Autodesk Inventor part; units mm, degrees
ref_plane "YZ Plane" through (0, 0, 0) normal (1, 0, 0) x (0, 1, 0)
ref_plane "XZ Plane" through (0, 0, 0) normal (0, 1, 0) x (-1, 0, 0)
ref_plane "XY Plane" through (0, 0, 0) normal (0, 0, 1) x (1, 0, 0)
sketch "Sketch1" plane through (0, 0, 0) normal (1, 0, 0) x (0, 1, 0)
  line L0 (0, 0) -> (64, 0)
  line L1 (0, 0) -> (56, 0)
  line L2 (0, 0) -> (8, 0)
  line L3 (0, 0) -> (0, -95)
  line L4 (0, 0) -> (0, -82)
  line L5 (0, 0) -> (6, 0)
  line L6 (64, 0) -> (64, -13)
  line L7 (64, -13) -> (64, -22)
  line L8 (56, 0) -> (56, -13) construction
  line L9 (56, -22) -> (64, -22) construction
  line L10 (56, -22) -> (56, -95) construction
  line L11 (56, -95) -> (0, -95) construction
  line L12 (64, -22) -> (56, -22)
  line L13 (0, -95) -> (0, -107)
  line L14 (0, -107) -> (8, -107)
  line L15 (8, -107) -> (8, -95)
  line L16 (113.6296, 0) -> (-73.0224, 0)
  line L17 (0, -82) -> (56, -82) construction
  line L18 (8, -95) -> (8, -82)
  line L19 (56, -82) -> (8, -82)
  line L20 (56, -82) -> (56, -22)
  line L21 (8, -95) -> (0, -95)
  arc A0 (0, -85.7011) -> (56, -22) centre (-35.8458, 2.2766) ccw construction
  line L22 (0, -82) -> (0, -85.7011)
  line L23 (56, -22) -> (56, -30)
  line L24 (56, -13) -> (56, 0) construction
  arc A1 (0, -82) -> (54.4542, -13) centre (-35.8458, 2.2766) ccw construction
  line L25 (64, -13) -> (54.4542, -13)
  line L26 (56, -22) -> (56, 0) construction
  arc A2 (8, -82) -> (56, -22) centre (-35.8458, 2.2766) ccw
  line L27 (-35.8458, 2.2766) -> (-35.8458, 0)
  arc A3 (0, -82) -> (54.4542, -13) centre (-35.8458, 2.2766) ccw
  line L28 (8, -82) -> (0, -82)
  point P0 (-35.8458, 1.1383)
  point P1 (8, -82)
  point P2 (8, -82)
  dimension "d0" = 64
  dimension "d1" = 56
  dimension "d2" = 8
  dimension "d3" = 95
  dimension "d4" = 82
  dimension "d5" = 6
  dimension "d6" = 13
  dimension "d7" = 9
  dimension "d12" = 12
ref_plane "Work Plane3" through (0, 0, 0) normal (0, -1, 0) x (1, 0, 0)
sketch "Sketch3" plane through (0, 0, 0) normal (0, -1, 0) x (1, 0, 0)
  circle A0 centre (0, 0) radius 95
  circle A1 centre (0, -95) radius 11.9643
  circle A2 centre (82.2724, -47.5) radius 11.9643
  circle A3 centre (82.2724, 47.5) radius 11.9643
  circle A4 centre (0, 95) radius 11.9643
  circle A5 centre (-82.2724, 47.5) radius 11.9643
  circle A6 centre (-82.2724, -47.5) radius 11.9643
  dimension "d15" = 360
ref_plane "Work Plane1" through (0, 56, 0) normal (0, 1, 0) x (1, 0, 0)
extrude "Extrusion2" add sketch "Sketch3" against normal blind 8 contours A3 A0 | A0 A3 | A2 A0 | A0 A2 | A4 A0 | A0 A4 | A1 A0 | A0 A1 | A5 A0 | A0 A5 | A6 A0 | A0 A6
revolve "Revolution2" add sketch "Sketch1" angle 360 about axis through (0, 113.6296, 0) along (0, -1, 0) contours L0 L6 L25 A3 L3 | L28 L18 L21 L3 | A3 L25 L7 L12 A2 L28 | A2 L20 L19
sketch "Sketch5" plane through (0, 56, 0) normal (0, 1, 0) x (1, 0, 0)
  arc A0 (-75.6497, 57.4641) -> (-87.5902, 36.7825) centre (-82.2724, 47.5) ccw
  circle A1 centre (-82.2724, 47.5) radius 4
  circle A2 centre (-82.2724, -47.5) radius 4
  circle A3 centre (0, -95) radius 4
  circle A4 centre (82.2724, -47.5) radius 4
  circle A5 centre (82.2724, 47.5) radius 4
  circle A6 centre (0, 95) radius 4
  point P0 (0, 0)
  dimension "d20" = 8
  dimension "d23" = 360
extrude "Extrusion3" cut sketch "Sketch5" against normal blind 64
sketch "Sketch8" plane through (0, 64, 0) normal (0, 1, 0) x (1, 0, 0)
  circle A0 centre (0, 0) radius 13
  dimension "d39" = 26
extrude "Extrusion4" cut sketch "Sketch8" against normal blind 64
sketch "Sketch9" plane through (0, 56, 0) normal (0, 1, 0) x (1, 0, 0)
  circle A0 centre (0, 0) radius 82
  line L0 (0, 82) -> (67.9153, 82) construction
  line L1 (0, 82) -> (8, 82)
  line L2 (-82, 0) -> (82, 0)
  line L3 (8, 82) -> (8, 0)
  line L4 (8, 82) -> (-8, 82)
  line L5 (-8, 82) -> (-8, 0)
  line L6 (0, 0) -> (0, -42) construction
  line L7 (0, -42) -> (0, -61) construction
  circle A1 centre (0, -42) radius 12 construction
  circle A2 centre (0, -42) radius 8 construction
  circle A3 centre (0, -61) radius 12 construction
  circle A4 centre (0, -61) radius 8 construction
  line L8 (-12, -61) -> (-12, -42)
  line L9 (12, -61) -> (12, -42)
  line L10 (-12, -61) -> (12, -61) construction
  line L11 (-12, -42) -> (12, -42) construction
  arc A5 (-12, -61) -> (12, -61) centre (0, -61) ccw
  arc A6 (12, -42) -> (-12, -42) centre (0, -42) ccw
  arc A7 (8, -42) -> (-8, -42) centre (0, -42) ccw
  arc A8 (-8, -61) -> (8, -61) centre (0, -61) ccw
  line L12 (-8, -61) -> (-8, -42)
  line L13 (8, -61) -> (8, -42)
  point P0 (8, 81.6088)
  point P1 (-8, 81.6088)
  dimension "d42" = 8
  dimension "d43" = 16
  dimension "d44" = 42
  dimension "d45" = 19
  dimension "d46" = 24
  dimension "d47" = 16
  dimension "d48" = 24
  dimension "d49" = 16
extrude "Extrusion5" cut sketch "Sketch9" against normal blind 56 contours L2 A0 | A0 L5 L2 | L2 L3 A0
revolve "Revolution3" add sketch "Sketch1" angle 360 about axis through (0, 113.6296, 0) along (0, -1, 0) contours A3 L25 L7 L12 A2 L28
sketch "Sketch10" plane through (0, 56, 61) normal (0, 1, 0) x (1, 0, 0)
  circle A0 centre (0, 0) radius 8
  arc A1 (12, 19) -> (-12, 19) centre (0, 19) ccw
  circle A2 centre (0, 19) radius 8
  line L0 (-8, 0) -> (-8, 19)
  line L1 (8, 0) -> (8, 19)
  arc A3 (-12, 0) -> (12, 0) centre (0, 0) ccw
  line L2 (0, 0) -> (0, 19)
  line L3 (-8, 0) -> (8, 0)
  point P0 (0, 61)
  dimension "d54" = 16
  dimension "d55" = 16
extrude "Extrusion6" cut sketch "Sketch10" against normal blind 56
sketch "Sketch11" plane through (8, 56, -20.4939) normal (1, 0, 0) x (0, 0, -1)
  point P0 (-20.4939, -56)
sketch "Sketch12" plane through (0, 56, 0) normal (0, 1, 0) x (1, 0, 0)
  arc A0 (8, 81.6088) -> (-8, 81.6088) centre (0, 0) ccw
  line L0 (0, 82) -> (-26.239, 82)
  line L1 (-26.239, 82) -> (20.0179, 82)
  line L2 (8, 81.6088) -> (8, 82)
  line L3 (-8, 81.6088) -> (-8, 82)
  circle A1 centre (0, 0) radius 82
extrude "Extrusion7" add sketch "Sketch12" against normal blind 56 contours A0 L1 L2 | A0 L3 L0
sketch "Sketch13" plane through (8, 56, -20.4939) normal (1, 0, 0) x (0, 0, -1)
  line L0 (61.4732, -0.0625) -> (61.5061, -10.0624)
  line L1 (61.5061, 0) -> (61.5061, -48)
  line L2 (61.5061, -10.0624) -> (50.5062, -10.0986)
  circle A0 centre (50.5062, -10.0986) radius 4
  point P0 (-20.4939, -56)
  dimension "d60" = 10
  dimension "d61" = 11
  dimension "d62" = 8
extrude "Extrusion8" cut sketch "Sketch13" against normal blind 56
properties part number "Bai_11"
Can you work these out from the model? Positions are in its coordinate system, mm. A direction names the side the tool comes from. Give positions to 0.01 mm unless a question says otherwise; leave off trailing zeros. Write item = value, one per line. Start each with the question number.
1. For pin 1 (17.5 mm diameter, centred on x = -2, z = -51, fed in from +Y); pin 2 (5 mm diameter, centred on x = -82.27, z = 47.5, fed in from -Y); pin 3 (1 mm diameter, centred on x = -61, z = 41, fed in from +Y); pin 4 (6 mm diameter, centred on y = 18, z = -69.5, fed in from -X), each with a flat end and sliding along its axis, tell me the tip position at first contact or that it passes through.
2. On a 3-axis mill with a long thin cutter (end or side, diameter ignored), from which of +Z, -Z, +X, -X, +Y, -Y can I reach the whole of each face in a straight line? I mean faces 4 (the face through (8, 22, -38)), 5 (the face through (-9.5, 64, -9.5)), 6 (the face through (-21.477, 59.944, 4.769)). Say none if no direction works.
3. Thinking about a two-plate mould opening in Z: for faces 1 (the face through (8, 45, -65)), 2 (the face through (92.77, 3.94, 53.24)), 3 (the face through (47.957, 3.944, 82.007)), which applies, released by +Z, released by -Z, zero draft, split by the parting line, or undercut?
4. Please list where these lines run through material, in increasing order: line 1 (Z direction, x = -0.5, y = 61.5); line 2 (X direction, y = 4, z = 95); line 3 (X direction, y = 45, z = 52).
5. Imagine slicing it at A-A (y = 11). Count the separate pieces of the cut face and the enclosed holes in it, and give its area (3 significant figures).
Worked answers:
q1.pin_1 = 56
q1.pin_2 = through
q1.pin_3 = 22.11
q1.pin_4 = -38.17
q2.face_4 = -Y
q2.face_5 = +Z, -Z, +X, -X, +Y
q2.face_6 = +Y
q3.face_1 = zero draft
q3.face_2 = undercut
q3.face_3 = released by +Z
q4.line_1 = -21.99 to -12.99, 12.99 to 21.99
q4.line_2 = -11.96 to -4, 4 to 11.96
q4.line_3 = -12 to -8, 8 to 12
q5.separate_pieces = 2
q5.enclosed_holes = 2
q5.area = 3,400 mm2
